from build123d import *

# Parameters (mm, degrees)
MODEL_R             = 1.449812935
MODEL_R_2           = 7.999917631
MODEL_W             = 3.6
MODEL_H             = 6.173462
BOSS_EXTRUDE1_DEPTH = 5.85


with BuildPart() as part:
    # Model → Boss-Extrude1 (new body)
    with BuildSketch(Plane.XY):
        with BuildLine():
            ThreePointArc((531.251426748, 585.073190054), (533.909979714, 591.869304693), (540.677443159, 594.599966993))
            Line((540.677443159, 594.599966993), (568.674763139, 594.599966993))
            ThreePointArc((568.674763139, 594.599966993), (575.442226583, 591.869304693), (578.10077955, 585.073190054))
            add(Edge.make_bspline(
                [(578.10077955, 585.073190054), (577.425296665, 565.393042288), (567.160030567, 565.073190054)],
                knots=[0, 0, 0, 1, 1, 1], degree=2))
            Line((567.160030567, 565.073190054), (542.192175731, 565.073190054))
            add(Edge.make_bspline(
                [(531.251426748, 585.073190054), (531.926909632, 565.393042288), (542.192175731, 565.073190054)],
                knots=[0, 0, 0, 1, 1, 1], degree=2))
        make_face()
        with Locations((563.478415084, 571.273190054)):
            Circle(MODEL_R, mode=Mode.SUBTRACT)
        with Locations((541.283961295, 584.797511369)):
            Circle(MODEL_R_2, mode=Mode.SUBTRACT)
        with Locations((545.873791214, 571.273190054)):
            Circle(MODEL_R, mode=Mode.SUBTRACT)
        with Locations((568.068245003, 584.797511369)):
            Circle(MODEL_R_2, mode=Mode.SUBTRACT)
        with BuildLine():
            Line((560.676103149, 578.334674665), (560.676103149, 575.334674665))
            ThreePointArc((560.676103149, 575.334674665), (560.38320993, 574.627567884), (559.676103149, 574.334674665))
            Line((559.676103149, 574.334674665), (554.676103149, 574.334674665))
            Line((554.676103149, 574.334674665), (549.676103149, 574.334674665))
            ThreePointArc((549.676103149, 574.334674665), (548.968996368, 574.627567884), (548.676103149, 575.334674665))
            Line((548.676103149, 575.334674665), (548.676103149, 578.334674665))
            ThreePointArc((548.676103149, 578.334674665), (548.968996368, 579.041781446), (549.676103149, 579.334674665))
            Line((549.676103149, 579.334674665), (554.676103149, 579.334674665))
            Line((554.676103149, 579.334674665), (559.676103149, 579.334674665))
            ThreePointArc((559.676103149, 579.334674665), (560.38320993, 579.041781446), (560.676103149, 578.334674665))
        make_face(mode=Mode.SUBTRACT)
        with Locations((568.826370712, 571.273190054)):
            Rectangle(MODEL_W, MODEL_H, mode=Mode.SUBTRACT)
        with Locations((540.525835586, 571.273190054)):
            Rectangle(MODEL_W, MODEL_H, mode=Mode.SUBTRACT)
    extrude(amount=BOSS_EXTRUDE1_DEPTH)


solid = part.part
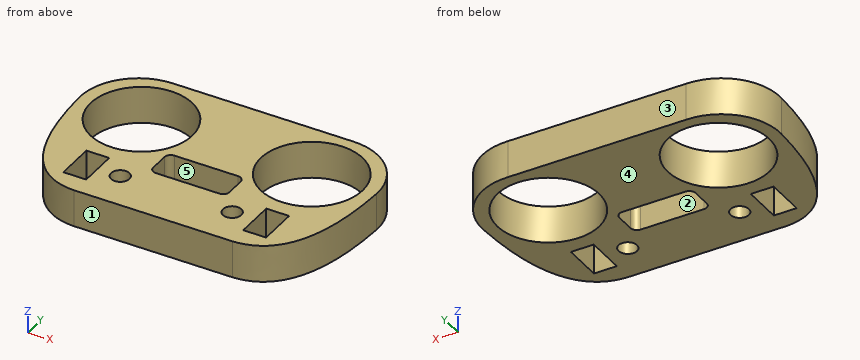
Could you check a few things on this model? Use its own coordinates, in mm. Face numbers are marked on the shaded views. A direction names the side the tool comes from. Give positions to 0.01 mm unless a question says otherwise; leave off trailing zeros. Order: outer loops, then holes, each group sorted by start corner. A loop starts at its lowest first (then second) coordinate and runs counter-clockwise, first axis right, second up. Notation, with made-up numbers: (0.25, 20) - (11.25, 20) arc R32 cw to (11.25, 49) - close; hole circle Ø8 at (75.5, 65.5). An arc over 180 degrees is marked (long way). Return JSON: item names as keys, results as strings. Group by question number.
Q1. Will these pins go through, and if not, where does the flat tip stop? pin 1 Ø3.5 at (y, z) = (577.5, 4.5) entering from +X; pin 2 Ø3.5 at (y, z) = (576.5, 4.5) entering from -X; pin 3 Ø1.8 at (x, z) = (553.5, 3.5) entering from +Y.
Q2. Thinking about a two-plate mould opening in Y: for the marked faces 1, 2 and 3, which applies, pulls with the +Y half, pulls with the -Y half, needs draft (parallel to the pull), parting line crosses it, or undercut?
Q3. Suppose I cut it at D-D, the plane z = 1.45. State how many separate pieces and enclosed holes the cut face has, and give its area (3 significant figures).
Q4. Please list where these lines run through material, in increasing order: line 1 along Y through (x, z) = (558, 3.7); line 2 along X through (y, z) = (588.5, 1.9); line 3 along Y through (x, z) = (546, 3.7). Write a range as [from, to].
Q5. Which directions (+Z, -Z, +X, -X, +Y, -Y) give clear straight access to the entire face, cutting with the end or side of a thin tool? Please do the marked faces 4 and 5.
Q6. Suppose I cut it at A-A, the plane x = 551.5. Please give me the cut outline in (y, z), and give its area (3 significant figures).
Q7. Suppose I cut it at B-B, the plane y = 586.75. Please give me the cut outline in (x, z), and give its area (3 significant figures).
Q8. Suppose I cut it at C-C, the plane x = 546. Please give me the cut outline in (y, z).
Resolved:
{
 "1": {"pin 1": "stops at x = 577.64", "pin 2": "stops at x = 531.86", "pin 3": "stops at y = 594.6"},
 "2": {"face 1": "pulls with the -Y half", "face 2": "undercut", "face 3": "pulls with the +Y half"},
 "3": {"separate pieces": "1", "enclosed holes": "7", "area": "744 mm2"},
 "4": {"line 1": "y = [565.07, 574.33], [579.33, 594.6]", "line 2": "x = [531.79, 534.19], [548.38, 560.98], [575.16, 577.57]", "line 3": "y = [565.07, 569.83], [572.72, 578.34], [591.26, 594.6]"},
 "5": {"face 4": "-Z, +X, -X, +Y, -Y", "face 5": "+Z, -Z"},
 "6": {"outline": "(565.07, 0) - (574.33, 0) - (574.33, 5.85) - (565.07, 5.85) - close; (579.33, 0) - (594.6, 0) - (594.6, 5.85) - (579.33, 5.85) - close", "area": "143 mm2"},
 "7": {"outline": "(531.35, 0) - (533.53, 0) - (533.53, 5.85) - (531.35, 5.85) - close; (549.04, 0) - (560.31, 0) - (560.31, 5.85) - (549.04, 5.85) - close; (575.83, 0) - (578.01, 0) - (578.01, 5.85) - (575.83, 5.85) - close", "area": "91.4 mm2"},
 "8": {"outline": "(565.07, 0) - (569.83, 0) - (569.83, 5.85) - (565.07, 5.85) - close; (572.72, 0) - (578.34, 0) - (578.34, 5.85) - (572.72, 5.85) - close; (591.26, 0) - (594.6, 0) - (594.6, 5.85) - (591.26, 5.85) - close"}
}
